Here's how the part is built. I have some questions about the finished solid (model axes, mm). Give positions to 0.01 mm unless a question says otherwise; leave off trailing zeros. Order: outer loops, then holes, each group sorted by start corner. A loop starts at its lowest first (then second) coordinate and runs counter-clockwise, first axis right, second up.
from build123d import *

# Parameters (mm, degrees)
SKETCH1_W           = 76.2
SKETCH1_H           = 127
BOSS_EXTRUDE1_DEPTH = 6.35
SKETCH3_R           = 3.175
SKETCH3_W           = 25.493937525
SKETCH3_H           = 25.320509378
SKETCH3_W_2         = 25.4
CUT_EXTRUDE2_DEPTH  = 6.35


with BuildPart() as part:
    # Sketch1 → Boss-Extrude1 (new body)
    with BuildSketch(Plane.XY):
        with Locations((38.1, 63.5)):
            Rectangle(SKETCH1_W, SKETCH1_H)
    extrude(amount=BOSS_EXTRUDE1_DEPTH)

    # Sketch3 → Cut-Extrude2 (cut)
    with BuildSketch(Plane.XY.offset(6.35)):
        with Locations((38.1, 63.5)):
            Circle(SKETCH3_R)
        with Locations((37.83985778, 88.939745311)):
            Rectangle(SKETCH3_W, SKETCH3_H)
        with Locations((38.1, 38.060254689)):
            Rectangle(SKETCH3_W_2, SKETCH3_H)
    extrude(amount=-CUT_EXTRUDE2_DEPTH, mode=Mode.SUBTRACT)


solid = part.part
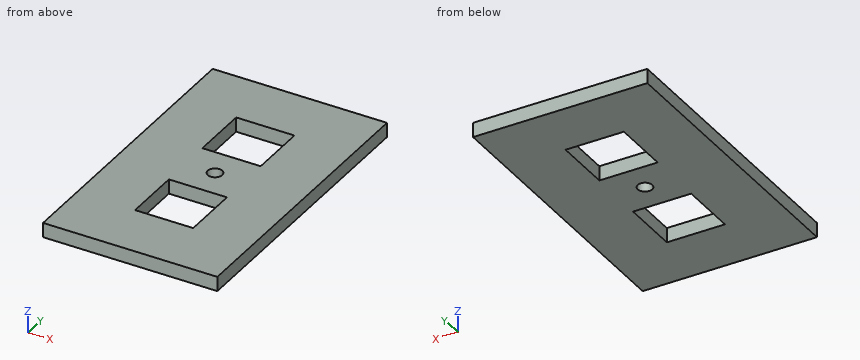
Q1. If we section it at B-B on x = 38.1: Give the number of separate pieces and of enclosed holes in the cut face, plus the area to 3 significant figures.
Filled sheet:
separate pieces: 4
enclosed holes: 0
area: 445 mm2
Q2. If we section it at D-D on y = 63.5: List the corners of the cut face in (x, z) for me (3 decimals).
Filled sheet:
outline: (0, 0) - (34.925, 0) - (34.925, 6.35) - (0, 6.35) - close; (41.275, 0) - (76.2, 0) - (76.2, 6.35) - (41.275, 6.35) - close
Q3. I need wall thicknesses on L1, parallel to Y at x = 38.1, z = 4.25 (1 decimal); L2, parallel to X at y = 85.5, z = 5.25; L3, parallel to Y at x = 40, z = 2.25. Which ranges of each line are inside material? Lowest first, please.
Filled sheet:
L1: y = 0 to 25.4, 50.7 to 60.3, 66.7 to 76.3, 101.6 to 127
L2: x = 0 to 25.09, 50.59 to 76.2
L3: y = 0 to 25.4, 50.72 to 60.96, 66.04 to 76.28, 101.6 to 127
Q4. If we section it at A-A on y = 95.5: List the corners of the cut face in (x, z) for me, plus the area to 3 significant figures.
Filled sheet:
outline: (0, 0) - (25.09, 0) - (25.09, 6.35) - (0, 6.35) - close; (50.59, 0) - (76.2, 0) - (76.2, 6.35) - (50.59, 6.35) - close
area: 322 mm2
